from build123d import *

# Parameters (mm, degrees)
SKETCH1_R           = 16.51
BOSS_EXTRUDE2_DEPTH = 20
SKETCH2_R           = 13.6906
BOSS_EXTRUDE3_DEPTH = 32.512
SKETCH3_R           = 1.5
CUT_EXTRUDE1_DEPTH  = 6.35
SKETCH4_R           = 4.953
BOSS_EXTRUDE4_DEPTH = 2.54
SKETCH5_R           = 2.5
BOSS_EXTRUDE5_DEPTH = 10.16
SKETCH6_R           = 5
BOSS_EXTRUDE6_DEPTH = 2
SKETCH7_R           = 1.143
BOSS_EXTRUDE7_DEPTH = 3.048
CUT_EXTRUDE2_DEPTH  = 8.382


with BuildPart() as part:
    # Sketch1 → Boss-Extrude2 (new body)
    with BuildSketch(Plane(origin=(0, 0, 0), x_dir=(0, 0, -1), z_dir=(1, 0, 0))):
        Circle(SKETCH1_R)
    extrude(amount=BOSS_EXTRUDE2_DEPTH)

    # Sketch2 → Boss-Extrude3 (add)
    with BuildSketch(Plane.ZY):
        Circle(SKETCH2_R)
    extrude(amount=BOSS_EXTRUDE3_DEPTH)

    # Sketch3 → Cut-Extrude1 (cut)
    with BuildSketch(Plane(origin=(20, 0, 0), x_dir=(0, 0, -1), z_dir=(1, 0, 0))):
        with Locations((0, 13.51)):
            Circle(SKETCH3_R)
        with Locations((11.75, -6.841596989)):
            Circle(SKETCH3_R)
        with Locations((-11.75, -6.841596989)):
            Circle(SKETCH3_R)
    extrude(amount=-CUT_EXTRUDE1_DEPTH, mode=Mode.SUBTRACT)

    # Sketch4 → Boss-Extrude4 (add)
    with BuildSketch(Plane(origin=(20, 0, 0), x_dir=(0, 0, -1), z_dir=(1, 0, 0))):
        with Locations((0, -6.604)):
            Circle(SKETCH4_R)
    extrude(amount=BOSS_EXTRUDE4_DEPTH)

    # Sketch5 → Boss-Extrude5 (add)
    with BuildSketch(Plane(origin=(22.54, 0, 0), x_dir=(0, 0, -1), z_dir=(1, 0, 0))):
        with Locations((0, -6.604)):
            Circle(SKETCH5_R)
    extrude(amount=BOSS_EXTRUDE5_DEPTH)

    # Sketch6 → Boss-Extrude6 (add)
    with BuildSketch(Plane.ZY.offset(32.512)):
        Circle(SKETCH6_R)
    extrude(amount=BOSS_EXTRUDE6_DEPTH)

    # Sketch7 → Boss-Extrude7 (add)
    with BuildSketch(Plane.ZY.offset(34.512)):
        Circle(SKETCH7_R)
    extrude(amount=BOSS_EXTRUDE7_DEPTH)

    # Sketch8 → Cut-Extrude2 (cut)
    with BuildSketch(Plane(origin=(32.7, 0, 0), x_dir=(0, 0, -1), z_dir=(1, 0, 0))):
        with BuildLine():
            Line((2, -8.104), (-2, -8.104))
            ThreePointArc((-2, -8.104), (0, -9.104), (2, -8.104))
        make_face()
    extrude(amount=-CUT_EXTRUDE2_DEPTH, mode=Mode.SUBTRACT)


solid = part.part
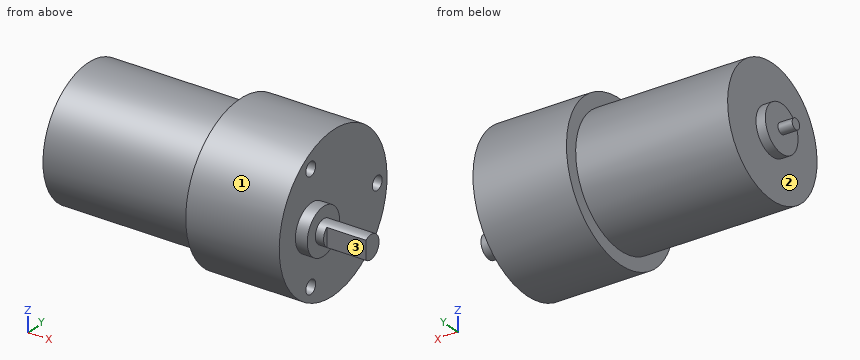
Model file for the job. Use its own axes, mm. Face numbers are marked on the shaded views. A direction names the side the tool comes from. Coordinates: 2 decimals unless noted, no trailing zeros. Write each loop counter-clockwise with the first axis right and the second up, starting at its lowest first coordinate (ties: lowest second). Pieces come first, ordered by that corner, then holes. Notation, with made-up numbers: (75, 34) - (129, 34) arc R24 cw to (129, 55) - close; hole circle Ø7 at (8.5, 61.25). An arc over 180 degrees is marked (long way). Write each question's results on one line, items separated by ' | '. Start each with the question number.
1) Cut at A-A (y = 0). Write the cut outline in (x, z).
2) Flat gauge pins, fed straight in: P1, Ø5, axis at y = -8, z = 9, coming from the +X side; P2, Ø8, axis at x = -9.5, y = -7.5, coming from the -Z side; P3, Ø2, axis at y = -7.5, z = 1.5, coming from the -X side; P4, Ø16.5, axis at y = -6, z = 2.5, coming from the +X side. Where does each tip first touch, or does it go through?
3) 3-axis set-ups, long thin cutter, end or side, ignore diameter. For the marked faces 1, 2 and 3: which of +Z, -Z, +X, -X, +Y, -Y reach the whole face in a straight line?
4) Cut at C-C (x = -17). Write the cut outline in (y, z).
5) Cut at D-D (y = -12.5). Write the cut outline in (x, z), then the cut area to 3 significant figures.
6) Probe line 1 along Y through (x, z) = (17, 0); line 2 along Z through (x, y) = (19, -6); line 3 along X through (y, z) = (10, -5.5). List the from-to ranges inside material, lowest first. Write a range as from..to.
Returned:
1) outline: (-37.56, -1.14) - (-34.51, -1.14) - (-34.51, -5) - (-32.51, -5) - (-32.51, -13.69) - (0, -13.69) - (0, -16.51) - (20, -16.51) - (20, 16.51) - (0, 16.51) - (0, 13.69) - (-32.51, 13.69) - (-32.51, 5) - (-34.51, 5) - (-34.51, 1.14) - (-37.56, 1.14) - close
2) P1: x = 20 | P2: z = -13.24 | P3: x = -32.51 | P4: x = 32.7
3) face 1: +X, -X | face 2: -X | face 3: +Z, -Z, +X, -Y
4) outline: circle Ø27.38 at (0, 0)
5) outline: (-32.51, -5.58) - (0, -5.58) - (0, -10.79) - (20, -10.79) - (20, 10.79) - (0, 10.79) - (0, 5.58) - (-32.51, 5.58) - close | area: 795 mm^2
6) line 1: -16.51..12.01, 15.01..16.51 | line 2: -15.38..-12.99, -10.51..10.51, 12.99..15.38 | line 3: -32.51..20
